Drawing for the job (mm, zero at the part's lowest x, y, z). A direction names the side the tool comes from. Give positions to 0.01 mm unless a question says otherwise; leave off trailing zeros. Order: outer loops, then holes, each group sorted by start corner. A loop starts at its lowest first (then second) coordinate and runs counter-clockwise, first axis right, second up. Notation, with made-up numbers: (19.25, -1.75) - (38.25, -1.75) arc R9 cw to (38.25, 6.25) - close; hole circle Ø10 at (-24.5, 2). An arc over 180 degrees is marked (long way). Use a Markdown table: item, result. Add a question column.
(1) Slice it at A-A (z = 5). Write the cut outline in (x, y) (1 decimal).
(2) Slice it at D-D (x = 10.5). Write the cut outline in (y, z).
(3) Flat gauge pins, fed straight in: pin 1 (4 mm diameter, centred on x = 7.5, z = 6, fed in from +Y); pin 2 (5 mm diameter, centred on x = 11, z = 8, fed in from -Y); pin 3 (0.5 mm diameter, centred on y = 5.5, z = 8.5, fed in from -X); pin 4 (1.8 mm diameter, centred on y = 12.5, z = 7, fed in from -X). Where does each tip first touch, or does it go through?
(4) Wall check: line 1 (X direction, y = 1.2, z = 5); line 2 (Z direction, x = 12, y = 10); line 3 (Y direction, x = 10.05, z = 5). Give the ranges that are in metal, low to high.
(5) Slice it at C-C (x = 5). Write the cut outline in (y, z) (1 decimal).
(6) Slice it at B-B (y = 10). Write the cut outline in (x, z).
(7) Which spindle directions (+Z, -Z, +X, -X, +Y, -Y) get a long thin tool onto all of the face, cutting with end or side? Do the marked faces 1, 2, 3 and 4. Say none if no direction does.
(8) Mould opens along Z. For the marked faces 5, 6, 7 and 8 say: +Z half, -Z half, draft (parallel to the pull), parting line (faces both ways), or undercut.
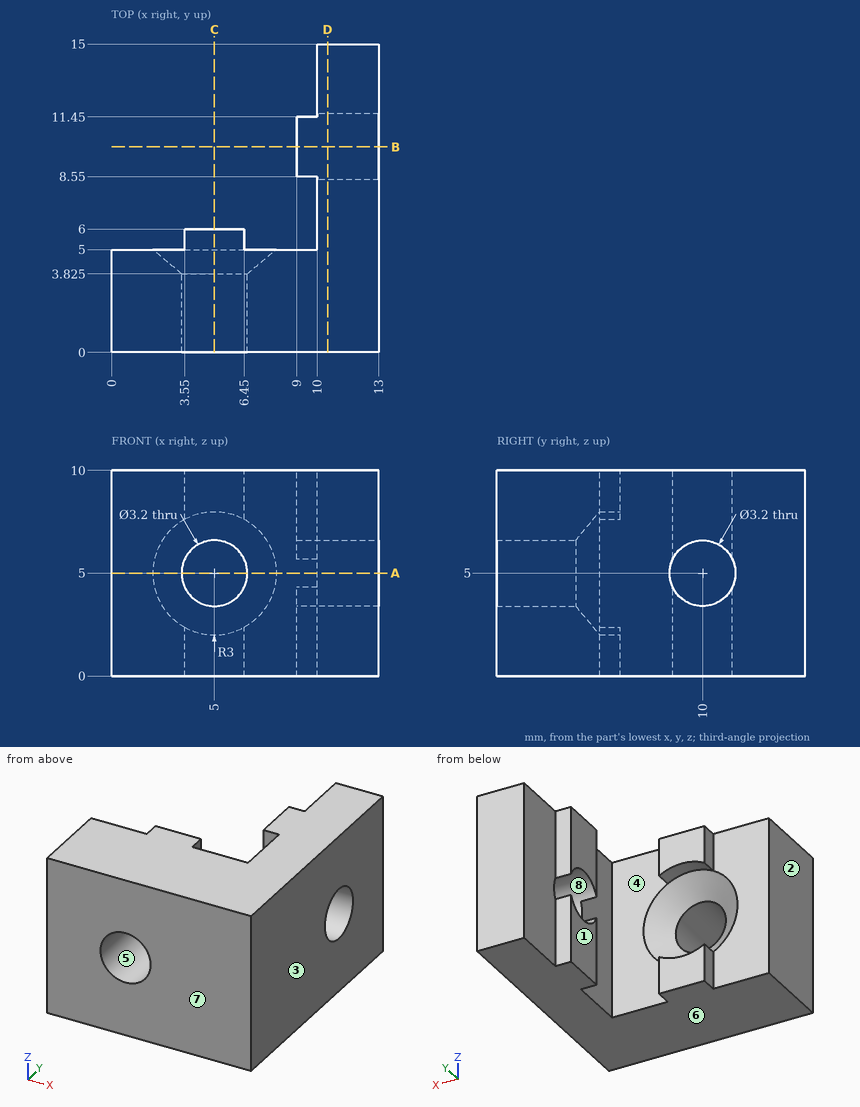
Solution:
| question | item | result |
|---|---|---|
| 1 | outline | (0, 0) - (3.4, 0) - (3.4, 3.8) - (2, 5) - (0, 5) - close; (6.6, 0) - (13, 0) - (13, 8.4) - (10, 8.4) - (10, 5) - (8, 5) - (6.6, 3.8) - close; (10, 11.6) - (13, 11.6) - (13, 15) - (10, 15) - close |
| 2 | outline | (0, 0) - (15, 0) - (15, 10) - (0, 10) - close; hole circle Ø3.2 at (10, 5) |
| 3 | pin 1 | y = 11.45 |
| 3 | pin 2 | y = 0 |
| 3 | pin 3 | x = 3.55 |
| 3 | pin 4 | x = 10 |
| 4 | line 1 | 0 to 3.4, 6.6 to 13 |
| 4 | line 2 | 0 to 3.4, 6.6 to 10 |
| 4 | line 3 | 0 to 8.4, 11.6 to 15 |
| 5 | outline | (0, 0) - (6, 0) - (6, 2) - (5, 2) - (3.8, 3.4) - (0, 3.4) - close; (0, 6.6) - (3.8, 6.6) - (5, 8) - (6, 8) - (6, 10) - (0, 10) - close |
| 6 | outline | (9, 0) - (13, 0) - (13, 3.4) - (9, 3.4) - close; (9, 6.6) - (13, 6.6) - (13, 10) - (9, 10) - close |
| 7 | face 1 | +Z, -Z, -X, +Y |
| 7 | face 2 | +Z, -Z, -X, +Y, -Y |
| 7 | face 3 | +Z, -Z, +X, +Y, -Y |
| 7 | face 4 | +Z, -Z |
| 8 | face 5 | undercut |
| 8 | face 6 | -Z half |
| 8 | face 7 | draft |
| 8 | face 8 | undercut |
